```python
from build123d import *

# Parameters (mm, degrees)
L_ANGLE_EQUAL_60X60X6_6_DEPTH = 1670
SKETCH14_R                    = 4
CUT_EXTRUDE1_DEPTH            = 1673.1542991
CHAMFER1_SIZE                 = 5.5
SKETCH18_R                    = 4
CUT_EXTRUDE2_DEPTH            = 1673.1542991
LPATTERN1_COUNT               = 5
LPATTERN1_PITCH               = 400
LPATTERN1_COUNT_DIR2          = 5
LPATTERN1_PITCH_DIR2          = 400


with BuildPart() as part:
    # Sketch17 → L angle (equal) 60X60X6(6) (new body)
    with BuildSketch(Plane(origin=(0, 0, 0), x_dir=(0, 0, -1), z_dir=(1, 0, 0))):
        with BuildLine():
            Line((0, 60), (0, 0))
            Line((0, 0), (60, 0))
            ThreePointArc((60, 0), (58.242640687, 4.242640687), (54, 6))
            Line((54, 6), (14, 6))
            ThreePointArc((14, 6), (8.343145751, 8.343145751), (6, 14))
            Line((6, 14), (6, 54))
            ThreePointArc((6, 54), (4.242640687, 58.242640687), (0, 60))
        make_face()
    extrude(amount=L_ANGLE_EQUAL_60X60X6_6_DEPTH)

    # Sketch14 → Cut-Extrude1 (cut, through all)
    with BuildSketch(Plane.XY):
        with Locations((65, 30)):
            Circle(SKETCH14_R)
        with Locations((1605, 30)):
            Circle(SKETCH14_R)
        with Locations((1650, 30)):
            Circle(SKETCH14_R)
        with Locations((20, 30)):
            Circle(SKETCH14_R)
    extrude(amount=-CUT_EXTRUDE1_DEPTH, mode=Mode.SUBTRACT)

    # Chamfer1
    chamfer1_edges = [part.edges().sort_by_distance(p)[0] for p in [
        (16, 30, -6),
        (1646, 30, -6),
        (1601, 30, -6),
        (61, 30, -6),
    ]]
    chamfer(chamfer1_edges, length=CHAMFER1_SIZE)

    # Sketch18 → Cut-Extrude2 (cut, through all)
    with BuildSketch(Plane(origin=(0, 0, 0), x_dir=(-1, 0, 0), z_dir=(0, -1, 0))):
        with Locations(Location((-35, 30, 0), (0, 0, 90))):
            Circle(SKETCH18_R)
    cut_extrude2 = extrude(amount=-CUT_EXTRUDE2_DEPTH, mode=Mode.SUBTRACT)

    # LPattern1: Cut-Extrude2 5 × 5
    with Locations(*[(i * LPATTERN1_PITCH, -j * LPATTERN1_PITCH_DIR2, 0) for i in range(LPATTERN1_COUNT) for j in range(LPATTERN1_COUNT_DIR2) if (i, j) != (0, 0)]):
        add(cut_extrude2, mode=Mode.SUBTRACT)


solid = part.part
```
Could you check a few things on this model? Use its own coordinates, in mm. A direction names the side the tool comes from. Round coordinates to 2 decimals unless told otherwise and drop trailing zeros. Loops run counter-clockwise (first coordinate to the right, second up) from the corner with the lowest first, then second, coordinate; pieces in that order, holes last. Notation, with made-up numbers: (88, 21) - (95, 21) arc R32 ccw to (95, 58) - close; hole circle Ø6 at (66, -28). An arc over 180 degrees is marked (long way). Answer in a Markdown table with one row per item. Add a question column.
(1) I'm going to push flat-ended pins straight in: pin 1 (10.5 mm diameter, centred on x = 1605, y = 30, fed in from +Z); pin 2 (13 mm diameter, centred on x = 65, y = 30, fed in from -Z); pin 3 (10 mm diameter, centred on x = 1446.5, z = -16, fed in from +Y); pin 4 (20 mm diameter, centred on x = 1175.5, z = -34, fed in from +Y). Where does each tip first touch, or does it pass through?
(2) If we section it at A-A (x = 1489): Please give me the cut outline in (y, z), plus the area to 3 significant figures.
(3) I need wall thicknesses on line 1 along Z through (x, y) = (1635, 1); line 2 along Y through (x, z) = (1650, -0.1); line 3 along Z through (x, y) = (374.5, 13.5). Which ranges of each line are inside material? Lowest first, please.
(4) For faces 1 (the face through (823, 34, -6)), 2 (the face through (0, 17, -5)), which set-ups out of +Z, -Z, +X, -X, +Y, -Y let a thin tool reach every point of the face, with its end or its side?
Model answer:
| question | item | result |
|---|---|---|
| 1 | pin 1 | stops at z = 0 |
| 1 | pin 2 | stops at z = -3 |
| 1 | pin 3 | stops at y = 6.58 |
| 1 | pin 4 | stops at y = 6 |
| 2 | outline | (0, -60) arc R6 ccw to (6, -54) - (6, -14) arc R8 cw to (14, -6) - (54, -6) arc R6 ccw to (60, 0) - (0, 0) - close |
| 2 | area | 682 mm² |
| 3 | line 1 | z = -59.92 to -34, -26 to 0 |
| 3 | line 2 | y = 0 to 26, 34 to 60 |
| 3 | line 3 | z = -6.02 to 0 |
| 4 | face 1 | -Z, +X, -X, +Y |
| 4 | face 2 | +Z, -Z, -X, +Y, -Y |
